from build123d import *

# Parameters (mm, degrees)
SKETCH_1_W          = 17
SKETCH_1_H          = 6.237893195
SKETCH_1_R          = 1.75
EXTRUDE_1_DEPTH     = 4
SKETCH_1_H_2        = 6.200638702
EXTRUDE_1_2_DEPTH   = 4
SKETCH_3_R          = 10.75
SKETCH_3_R_2        = 1.75
EXTRUDE_3_DEPTH     = 2
SKETCH_4_R          = 6.5
CUT_EXTRUDE_1_DEPTH = 10
SKETCH_5_R          = 12.75
SKETCH_5_R_2        = 10.75
EXTRUDE_1_3_DEPTH   = 10
SKETCH_6_R          = 5.171558732
CUT_EXTRUDE_2_DEPTH = 2


with BuildPart() as part:
    # Sketch 1 → Extrude 1 (new body)
    with BuildSketch(Plane.XY):
        with Locations((0, -116.390757476)):
            Rectangle(SKETCH_1_W, SKETCH_1_H)
        with Locations((0, -116.802352716)):
            Circle(SKETCH_1_R, mode=Mode.SUBTRACT)
    extrude(amount=EXTRUDE_1_DEPTH)



with BuildPart() as body_2:
    # Sketch 1 → Extrude 1 2 (new body)
    with BuildSketch(Plane.XY):
        with Locations((0, -188.663897323)):
            Rectangle(SKETCH_1_W, SKETCH_1_H_2)
        with Locations((0, -188.764216674)):
            Circle(SKETCH_1_R, mode=Mode.SUBTRACT)
    extrude(amount=EXTRUDE_1_2_DEPTH)


with BuildPart() as part_1:
    add(part.part)

    add(body_2.part)  # Extrude 3 merges body 2
    # Sketch 3 → Extrude 3 (add)
    with BuildSketch(Plane.XY.offset(4)):
        with BuildLine():
            Line((-8.5, -113.271810879), (8.5, -113.271810879))
            Line((8.5, -113.271810879), (8.5, -121.50085412))
            ThreePointArc((8.5, -121.50085412), (32.236701024, -152.596752449), (8.5, -183.692650779))
            Line((8.5, -183.692650779), (8.5, -191.764216674))
            Line((8.5, -191.764216674), (-8.5, -191.764216674))
            Line((-8.5, -191.764216674), (-8.5, -183.692650779))
            ThreePointArc((-8.5, -183.692650779), (-32.236701024, -152.596752449), (-8.5, -121.50085412))
            Line((-8.5, -121.50085412), (-8.5, -113.271810879))
        make_face()
        with Locations((0, -172.399709936)):
            Circle(SKETCH_3_R, mode=Mode.SUBTRACT)
        with Locations((0, -188.764216674)):
            Circle(SKETCH_3_R_2, mode=Mode.SUBTRACT)
        with Locations((0, -116.802352716)):
            Circle(SKETCH_3_R_2, mode=Mode.SUBTRACT)
    extrude(amount=EXTRUDE_3_DEPTH)

    # Sketch 4 → Cut-Extrude 1 (cut)
    with BuildSketch(Plane.XY.offset(6)):
        with Locations((0, -152.596752449)):
            Circle(SKETCH_4_R)
    extrude(amount=-CUT_EXTRUDE_1_DEPTH, mode=Mode.SUBTRACT)

    # Sketch 5 → Extrude 1 3 (add)
    with BuildSketch(Plane.XY.offset(6)):
        with Locations((0, -172.399709936)):
            Circle(SKETCH_5_R)
        with Locations((0, -172.399709936)):
            Circle(SKETCH_5_R_2, mode=Mode.SUBTRACT)
    extrude(amount=EXTRUDE_1_3_DEPTH)

    # Sketch 6 → Cut-Extrude 2 (cut)
    with BuildSketch(Plane.XY.offset(6)):
        with Locations((0, -116.802352716)):
            Circle(SKETCH_6_R)
    extrude(amount=-CUT_EXTRUDE_2_DEPTH, mode=Mode.SUBTRACT)


solid = part_1.part
Part model, mm, in its own coordinate system. A direction names the side the tool comes from. Round coordinates to 2 decimals unless told otherwise and drop trailing zeros. Write each loop counter-clockwise with the first axis right and the second up, starting at its lowest first coordinate (ties: lowest second). Pieces come first, ordered by that corner, then holes. Notation, with made-up numbers: (-9, -22.5) - (42, -22.5) arc R23 ccw to (42, 16.5) - close; hole circle Ø11 at (82, -33). An arc over 180 degrees is marked (long way). Use CSV: the item, a comma, the result in double quotes.
Item 1: Wall check: L1, parallel to Y at x = 0, z = 1.2; L2, parallel to Y at x = 0, z = 5.6; L3, parallel to X at y = -172, z = 12.25. Give the ranges that are in metal, low to high.
Results list:
L1,"y = -191.76 to -190.51, -187.01 to -185.56, -119.51 to -118.55, -115.05 to -113.27"
L2,"y = -191.76 to -190.51, -187.01 to -183.15, -161.65 to -159.1, -146.1 to -121.97"
L3,"x = -12.74 to -10.74, 10.74 to 12.74"
Item 2: Tool access for faces 4 (the flat face through (-8.5, -117, 3)), 5 (the cylindrical face through (5.883, -183.711, 10.93)), 6 (the flat face through (0, -145, 4)), 7 (the flat face through (8.5, -189, 3)): list every direction of +Z, -Z, +X, -X, +Y, -Y with a clear straight run to the whole face (end or side of a thin tool).
Results list:
face 4,"+Z, -Z, -X, +Y"
face 5,"+Z"
face 6,"-Z, +X, -X"
face 7,"+Z, -Z, +X, -Y"
Item 3: Flat gauge pins, fed straight in: P1, Ø1.8, axis at y = -189.5, z = 3.5, coming from the -X side; P2, Ø6.5, axis at y = -189.5, z = 2.5, coming from the +X side; P3, Ø12, axis at x = -12, y = -127, coming from the -Z side; P4, Ø2, axis at x = 0, y = -188.76, coming from the -Z side. Where does each tip first touch, or does it go through?
Results list:
P1,"stops at x = -8.5"
P2,"stops at x = 8.5"
P3,"stops at z = 4"
P4,"passes through"
Item 4: Pull direction X, two halves, no side cores. Call faces 1 (the flat face through (0, -185.564, 2)), 2 (the flat face through (-8.5, -189, 3)), 3 (the flat face through (1, -115, 4)): pulls with the +X half, pulls with the -X half, needs draft (parallel to the pull), parting line crosses it, or undercut.
Results list:
face 1,"needs draft"
face 2,"pulls with the -X half"
face 3,"undercut"
Item 5: Slice it at B-B, the plane x = 0. Count the separate pieces of the cut face and the enclosed holes in it, then the cut area to 3 significant figures.
Results list:
separate pieces,"6"
enclosed holes,"0"
area,"125 mm²"
Item 6: Slice it at D-D, the plane y = -142. Write the cut outline in (x, z), then the cut area to 3 significant figures.
Results list:
outline,"(-30.45, 4) - (30.45, 4) - (30.45, 6) - (-30.45, 6) - close"
area,"122 mm²"
Item 7: Slice it at A-A, the plane y = -177. Write the cut outline in (x, z), then the cut area to 3 significant figures.
Results list:
outline,"(-21.06, 4) - (-9.72, 4) - (-9.72, 16) - (-11.89, 16) - (-11.89, 6) - (-21.06, 6) - close; (9.72, 4) - (21.06, 4) - (21.06, 6) - (11.89, 6) - (11.89, 16) - (9.72, 16) - close"
area,"88.9 mm²"
Item 8: Slice it at C-C, the plane z = 13.25. Write the cut outline in (x, y).
Results list:
outline,"circle Ø25.5 at (0, -172.4); hole circle Ø21.5 at (0, -172.4)"
